Part model, mm, in its own coordinate system. A direction names the side the tool comes from. Round coordinates to 2 decimals unless told otherwise and drop trailing zeros. Loops run counter-clockwise (first coordinate to the right, second up) from the corner with the lowest first, then second, coordinate; pieces in that order, holes last. Notation, with made-up numbers: M -7,80.5 L 26,80.5 A33 cw 26,111.5 Z; hole C -7,23 d4. An arc over 180 degrees is marked long. Put each result on its own line as item: value. Start each with the question number.
1) Pull direction X, two halves, no side cores. Call faces 6 (the flat face through (-1, 15, 26)), 7 (the flat face through (15.085, 14.79, 8.872)), 8 (the flat face through (-31.494, 14, 22)), 9 (the cylindrical face through (-7.81, 14.79, -1.73)): +X half, -X half, draft (parallel to the pull), parting line (faces both ways), or undercut.
2) Probe line 1 along X through (y, z) = (9, 0); line 2 along Y through (x, z) = (8, -15); line 3 along Z through (x, y) = (-1, 7). List the from-to ranges inside material, lowest first.
3) Which spindle directions (+Z, -Z, +X, -X, +Y, -Y) get a long thin tool onto all of the face, cutting with end or side? Do faces 1 (the flat face through (9, 0, 0)), 2 (the flat face through (-15.226, 14.79, 8.628)), 3 (the flat face through (9, 30, 0)), 4 (the flat face through (0, 15, -17.5)), 5 (the flat face through (-15.085, 14.79, -8.872)). Say none if no direction does.
4) Slice it at A-A on y = 16. Give the cut face in (x, z), then the cut area to 3 significant figures.
5) Slice it at C-C on z = -1. Give the cut face in (x, y), then the cut area to 3 significant figures.
6) Slice it at D-D on x = 17. Give the cut face in (y, z).
7) Slice it at B-B on x = 0. Give the cut face in (y, z).
8) Drop flat-ended pins along their axis: pin 1 Ø17.5 at (x, z) = (-4.5, -6.5) entering from +Y; pin 2 Ø4 at (x, z) = (-2.5, -5.5) entering from -Y; pin 3 Ø5 at (y, z) = (11.5, 0.5) entering from -X; pin 4 Ø6 at (y, z) = (15.5, 16) entering from +X. Give the stop position or say it passes through.
```python
from build123d import *

# Parameters (mm, degrees)
CROQUIS1_R              = 8
SALIENTE_EXTRUIR1_DEPTH = 30
CROQUIS2_W              = 62.253703669
CROQUIS2_H              = 47.910213751
SALIENTE_EXTRUIR2_DEPTH = 8.5


with BuildPart() as part:
    # Croquis1 → Saliente-Extruir1 (new body)
    with BuildSketch(Plane(origin=(0, 0, 0), x_dir=(1, 0, 0), z_dir=(0, 1, 0))):
        Polygon((20.207259422, 0), (10.103629711, 17.5), (-10.103629711, 17.5), (-20.207259422, 0), (-10.103629711, -17.5), (10.103629711, -17.5), align=None)
        with Locations(Location((0, 0, 0), (0, 0, 270))):
            Circle(CROQUIS1_R, mode=Mode.SUBTRACT)
    extrude(amount=SALIENTE_EXTRUIR1_DEPTH)

    # Croquis2 → Saliente-Extruir2 (add)
    with BuildSketch(Plane.XY.offset(17.5)):
        with Locations((-0.366655868, 14.825803959)):
            Rectangle(CROQUIS2_W, CROQUIS2_H)
    extrude(amount=SALIENTE_EXTRUIR2_DEPTH)


solid = part.part
```
Recorded:
1. face 6: draft
1. face 7: +X half
1. face 8: -X half
1. face 9: undercut
2. line 1: x = -20.21 to -8, 8 to 20.21
2. line 2: y = 0 to 30
2. line 3: z = -17.5 to -7.94, 7.94 to 26
3. face 1: -Z, +X, -X, -Y
3. face 2: -X, +Y, -Y
3. face 3: -Z, +X, -X, +Y
3. face 4: -Z, +X, -X, +Y, -Y
3. face 5: -Z, -X, +Y, -Y
4. outline: M -31.49,17.5 L -10.1,17.5 L -20.21,0 L -10.1,-17.5 L 10.1,-17.5 L 20.21,0 L 10.1,17.5 L 30.76,17.5 L 30.76,26 L -31.49,26 Z; hole C 0,0 d16
4. area: 1,390 mm2
5. outline: M -19.63,0 L -7.94,0 L -7.94,30 L -19.63,30 Z; M 7.94,0 L 19.63,0 L 19.63,30 L 7.94,30 Z
5. area: 702 mm2
6. outline: M -9.13,17.5 L 38.78,17.5 L 38.78,26 L -9.13,26 Z; M 0,-5.56 L 30,-5.56 L 30,5.56 L 0,5.56 Z
7. outline: M -9.13,17.5 L 0,17.5 L 0,8 L 30,8 L 30,17.5 L 38.78,17.5 L 38.78,26 L -9.13,26 Z; M 0,-17.5 L 30,-17.5 L 30,-8 L 0,-8 Z
8. pin 1: stops at y = 30
8. pin 2: stops at y = 0
8. pin 3: stops at x = -20.21
8. pin 4: stops at x = 30.76
